from build123d import *

# Parameters (mm, degrees)
CROQUIS1_W              = 300
CROQUIS1_H              = 300
SALIENTE_EXTRUIR1_DEPTH = 100
CROQUIS2_R              = 61.757793717
CROQUIS3_R              = 64.13831418
CROQUIS5_R              = 23.498626295


with BuildPart() as part:
    # Croquis1 → Saliente-Extruir1 (new body)
    with BuildSketch(Plane(origin=(0, 0, 0), x_dir=(1, 0, 0), z_dir=(0, 1, 0))):
        Rectangle(CROQUIS1_W, CROQUIS1_H)
    extrude(amount=SALIENTE_EXTRUIR1_DEPTH)

    # Barrer1: sweep along a curve in space
    with BuildLine() as barrer1_path:
        Line((79.719719639, 100, 0), (499.017442554, 807.657749643, 0))
    # Croquis2 → Barrer1 (sweep)
    with BuildSketch(Plane(origin=(0, 100, 0), x_dir=(1, 0, 0), z_dir=(0, 1, 0))):
        with Locations((79.719719639, 0)):
            Circle(CROQUIS2_R)
    sweep(path=barrer1_path.line)

    # Barrer2: sweep along a curve in space
    with BuildLine() as barrer2_path:
        Line((-82.576305282, 100, 0), (-442.652634805, 830.366298789, 0))
    # Croquis3 → Barrer2 (sweep)
    with BuildSketch(Plane(origin=(0, 100, 0), x_dir=(1, 0, 0), z_dir=(0, 1, 0))):
        with Locations((-82.576305282, 0)):
            Circle(CROQUIS3_R)
    sweep(path=barrer2_path.line)

    # Barrer4: sweep along a curve in space
    with BuildLine() as barrer4_path:
        Line((499.017442554, 807.657749643, 0), (499.017442554, 965.743179521, 0))
        ThreePointArc((499.017442554, 965.743179521, 0), (486.422687881, 1005.801110184, 0), (453.170648011, 1031.444189149, 0))
        Line((453.170648011, 1031.444189149, 0), (27.99293329, 1187.749316841, 0))
        ThreePointArc((27.99293329, 1187.749316841, 0), (4.508322897, 1192.045114145, 0), (-19.05406022, 1188.19870002, 0))
        Line((-395.546422858, 1057.899604458, 0), (-19.05406022, 1188.19870002, 0))
        ThreePointArc((-442.652634805, 991.749211651, 0), (-429.672653938, 1032.353613113, 0), (-395.546422858, 1057.899604458, 0))
        Line((-442.652634805, 830.366298789, 0), (-442.652634805, 991.749211651, 0))
    # Croquis5 → Barrer4 (sweep)
    with BuildSketch(Plane(origin=(0, 807.657749643, 0), x_dir=(1, 0, 0), z_dir=(0, 1, 0))):
        with Locations((499.017442554, 0)):
            Circle(CROQUIS5_R)
    sweep(path=barrer4_path.line)


solid = part.part
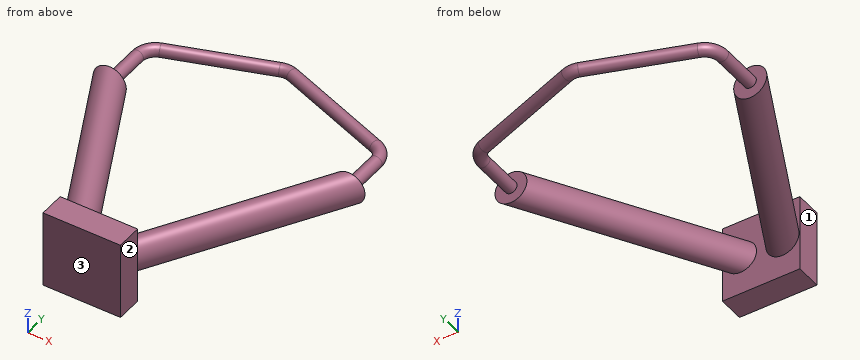
Here's how the part is built. I have some questions about the finished solid (model axes, mm). Face numbers are marked on the shaded views. A direction names the side the tool comes from. Coordinates: 2 decimals unless noted, no trailing zeros.
1) Which directions (+Z, -Z, +X, -X, +Y, -Y) give clear straight access to the entire face, cutting with the end or side of a thin tool? Please do the marked faces 1, 2 and 3.
Filled in:
face 1: +Z, -Z, -X, -Y
face 2: +Z, -Z, +X, -Y
face 3: +Z, -Z, +X, -X, -Y
2) I'm going to push flat-ended pins straight in: pin 1 (12 mm diameter, centred on y = 610, z = 22, fed in from -X); pin 2 (5 mm diameter, centred on x = 341.5, z = -19, fed in from -Y); pin 3 (5 mm diameter, centred on x = -175, z = -11, fed in from +Y). Where does each tip first touch, or does it pass through?
Filled in:
pin 1: stops at x = -397.83
pin 2: stops at y = 438.21
pin 3: stops at y = 1157.72
3) If I drill on line 1 (X direction, y = 532, z = -31); line 2 (X direction, y = 221, z = -43); line 3 (Y direction, x = -108, z = -115.5), over which ranges is the centre line in solid material (lowest first)?
Filled in:
line 1: x = -351.7 to -239.41, 282.27 to 389.1
line 2: x = -189.82 to -94.64, 107.09 to 195.74
line 3: y = 0 to 100
